The model under review builds one solid part; all positions refer to its coordinate system, in mm. A direction names the side the tool comes from. Give positions to 0.01 mm unless a question says otherwise; leave off trailing zeros. Order: outer loops, then holes, each group sorted by start corner. A loop starts at its lowest first (then second) coordinate and runs counter-clockwise, first axis right, second up.
```python
from build123d import *

# Parameters (mm, degrees)
CROQUIS1_W              = 12.5
CROQUIS1_H              = 32
SALIENTE_EXTRUIR1_DEPTH = 2
SALIENTE_EXTRUIR2_DEPTH = 21.9
CROQUIS5_W              = 1
CROQUIS5_H              = 15
SALIENTE_EXTRUIR4_DEPTH = 20
CROQUIS4_R              = 0.75
CORTAR_EXTRUIR1_DEPTH   = 5
REDONDEO1_R             = 1.5


with BuildPart() as part:
    # Croquis1 → Saliente-Extruir1 (new body)
    with BuildSketch(Plane(origin=(0, 111.467949425, 0), x_dir=(1, 0, 0), z_dir=(0, 1, 0))):
        with Locations((-9.702229413, -88.418391236)):
            Rectangle(CROQUIS1_W, CROQUIS1_H)
    extrude(amount=-SALIENTE_EXTRUIR1_DEPTH)

    # Croquis2 → Saliente-Extruir2 (add)
    with BuildSketch(Plane.XZ.offset(-109.467949425)):
        Polygon((-3.452229413, 101.418391236), (-5.452229413, 102.918391236), (-5.452229413, 73.918391236), (-3.452229413, 75.418391236), align=None)
    extrude(amount=SALIENTE_EXTRUIR2_DEPTH)

    # Croquis5 → Saliente-Extruir4 (add)
    with BuildSketch(Plane.XZ.offset(-109.467949425)):
        with Locations((-5.952229413, 88.418391236)):
            Rectangle(CROQUIS5_W, CROQUIS5_H)
    extrude(amount=SALIENTE_EXTRUIR4_DEPTH)

    # Croquis4 → Cortar-Extruir1 (cut, symmetric)
    with BuildSketch(Plane(origin=(0, 0, 88.418391236), x_dir=(0, -1, 0), z_dir=(0, 0, 1))):
        with Locations((-104.517949425, -3.452229413)):
            Circle(CROQUIS4_R)
        with Locations((-102.017949425, -3.452229413)):
            Circle(CROQUIS4_R)
        with Locations((-99.517949425, -3.452229413)):
            Circle(CROQUIS4_R)
        with Locations((-97.017949425, -3.452229413)):
            Circle(CROQUIS4_R)
        with Locations((-94.517949425, -3.452229413)):
            Circle(CROQUIS4_R)
    extrude(amount=CORTAR_EXTRUIR1_DEPTH, both=True, mode=Mode.SUBTRACT)

    # Redondeo1
    redondeo1_edges = [part.edges().sort_by_distance(p)[0] for p in [
        (-3.452229413, 110.467949425, 72.418391236),
        (-3.452229413, 110.467949425, 104.418391236),
    ]]
    fillet(redondeo1_edges, radius=REDONDEO1_R)


solid = part.part
```
1. Take a section at A-A (y = 92.5). Write out the cut boundary in (x, z), and give its area (3 significant figures).
2. Insertion check: pin 1 (6 mm diameter, centred on x = -13.5, z = 99.5, fed in from -Y); pin 2 (0.6 mm diameter, centred on x = -4, y = 94.5, fed in from -Z); pin 3 (0.8 mm diameter, centred on x = -6, z = 88, fed in from -Y); pin 4 (3 mm diameter, centred on y = 100, z = 84, fed in from +X). Each pin has a flat end and moves straight along its axis. Give the tip position at first contact, or say it passes through.
3. Take a section at C-C (x = -14.75). Write out the cut boundary in (y, z), and give its area (3 significant figures).
4. For faces 4 (the flat face through (-6, 100, 80.918)), 5 (the flat face through (-4.44, 98.67, 102.16)), 6 (the flat face through (-4.466, 98.671, 74.658)), 7 (the flat face through (-6.452, 100, 88)), list the 3-axis set-ups (+Z, -Z, +X, -X, +Y, -Y) from which the entire face can be reached by the end or side of a thin tool; tool diameter is ignored.
5. Take a section at D-D (z = 90). Write out the cut boundary in (x, y).
6. To check wall thickness, follow line 1 (X direction, y = 103.25, z = 96.5); line 2 (Z direction, x = -5.5, y = 101); line 3 (X direction, y = 99.25, z = 82.5). State the ranges of each line that lie inside material, in increasing order.
7. Draft analysis for pull direction Z (two halves, no side actions). For faces 1 (the flat face through (-4, 87.568, 89)), 2 (the flat face through (-6, 100, 95.918)), 3 (the cylindrical face through (-4.202, 94.534, 88.488)), state which applies: pulls with the +Z half, pulls with the -Z half, needs draft (parallel to the pull), parting line crosses it, or undercut.
8. Take a section at B-B (z = 80). Write out the cut boundary in (x, y).
Answer:
1. outline: (-6.45, 80.92) - (-5.45, 80.92) - (-5.45, 73.92) - (-3.45, 75.42) - (-3.45, 101.42) - (-5.45, 102.92) - (-5.45, 95.92) - (-6.45, 95.92) - close
1. area: 70.0 mm2
2. pin 1: stops at y = 109.47
2. pin 2: stops at z = 74.78
2. pin 3: stops at y = 89.47
2. pin 4: stops at x = -3.45
3. outline: (109.47, 72.42) - (111.47, 72.42) - (111.47, 104.42) - (109.47, 104.42) - close
3. area: 64.0 mm2
4. face 4: -Z, -X, -Y
4. face 5: +Z, +X, -Y
4. face 6: -Z, +X, -Y
4. face 7: +Z, -Z, -X, -Y
5. outline: (-15.95, 109.47) - (-6.45, 109.47) - (-6.45, 89.47) - (-5.45, 89.47) - (-5.45, 87.57) - (-3.45, 87.57) - (-3.45, 93.77) arc R0.75 cw to (-3.45, 95.27) - (-3.45, 96.27) arc R0.75 cw to (-3.45, 97.77) - (-3.45, 98.77) arc R0.75 cw to (-3.45, 100.27) - (-3.45, 101.27) arc R0.75 cw to (-3.45, 102.77) - (-3.45, 103.77) arc R0.75 cw to (-3.45, 105.27) - (-3.45, 111.47) - (-15.95, 111.47) - close
6. line 1: x = -5.45 to -3.45
6. line 2: z = 80.92 to 95.92
6. line 3: x = -6.45 to -3.45
7. face 1: needs draft
7. face 2: pulls with the +Z half
7. face 3: undercut
8. outline: (-15.95, 109.47) - (-5.45, 109.47) - (-5.45, 87.57) - (-3.45, 87.57) - (-3.45, 111.47) - (-15.95, 111.47) - close
